Check sheet for the drawn part. Datum: minimum x, y, z corner. Units: mm. Give positions to 0.01 mm unless a question says otherwise; leave off trailing zeros. Order: outer loops, then holes, each group sorted by start corner. A loop starts at its lowest first (then second) coordinate and runs counter-clockwise, first axis right, second up.
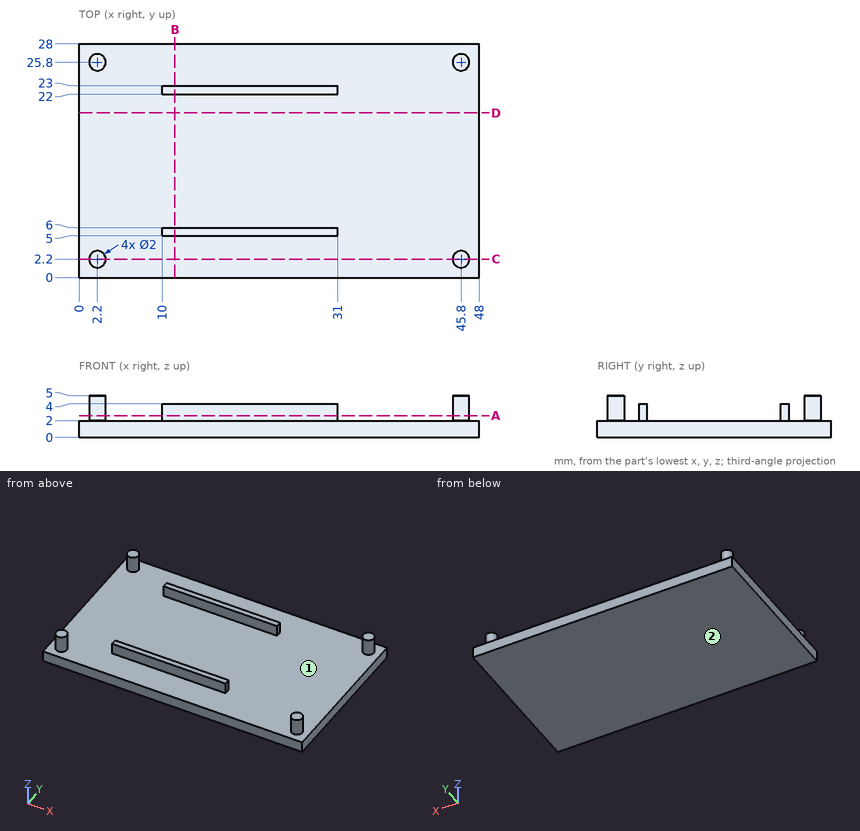
Item 1: Sectioned sample at D-D (y = 19.75). Enter the section's corners in (x, z).
Reported:
outline: (0, 0) - (48, 0) - (48, 2) - (0, 2) - close
Item 2: Draft check along X on the marked faces 1 and 2. Enter one of: released by +X, released by -X, zero draft, split by the parting line, or undercut.
Reported:
face 1: undercut
face 2: zero draft
Item 3: Gauge pin test, flat ends, axial feed: pin 1 (0.8 mm diameter, centred on y = 5.5, z = 3.5, fed in from +X); pin 2 (1 mm diameter, centred on x = 24.5, z = 3, fed in from -Y); pin 3 (10 mm diameter, centred on x = 25, y = 24, fed in from +Z). Record the tip position at first contact, or that the pin passes through.
Reported:
pin 1: stops at x = 31
pin 2: stops at y = 5
pin 3: stops at z = 4
Item 4: Sectioned sample at A-A (z = 2.6). Enter the section's corners in (x, y), and give its area (3 significant figures).
Reported:
outline: circle Ø2 at (2.2, 2.2); circle Ø2 at (2.2, 25.8); (10, 5) - (31, 5) - (31, 6) - (10, 6) - close; (10, 22) - (31, 22) - (31, 23) - (10, 23) - close; circle Ø2 at (45.8, 2.2); circle Ø2 at (45.8, 25.8)
area: 54.6 mm2
Item 5: Sectioned sample at B-B (x = 11.5). Enter the section's corners in (y, z).
Reported:
outline: (0, 0) - (28, 0) - (28, 2) - (23, 2) - (23, 4) - (22, 4) - (22, 2) - (6, 2) - (6, 4) - (5, 4) - (5, 2) - (0, 2) - close
Item 6: Sectioned sample at C-C (y = 2.2). Enter the section's corners in (x, z).
Reported:
outline: (0, 0) - (48, 0) - (48, 2) - (46.8, 2) - (46.8, 5) - (44.8, 5) - (44.8, 2) - (3.2, 2) - (3.2, 5) - (1.2, 5) - (1.2, 2) - (0, 2) - close
Item 7: Scan lines: L1, parallel to Y at x = 30.5, z = 3.25; L2, parallel to Z at x = 4.5, y = 22.5; L3, parallel to X at y = 26.25, z = 4.15. Record each from-to range of solid material in increasing order.
Reported:
L1: y = 5 to 6, 22 to 23
L2: z = 0 to 2
L3: x = 1.31 to 3.09, 44.91 to 46.69
